Part model, mm, in its own coordinate system. A direction names the side the tool comes from. Give positions to 0.01 mm unless a question says otherwise; leave off trailing zeros. Order: outer loops, then holes, each group sorted by start corner. A loop starts at its lowest first (then second) coordinate and runs counter-clockwise, first axis right, second up. Notation, with made-up numbers: M 24.5,-4.75 L 40.5,-4.75 A23 cw 40.5,9.25 Z; hole C 11,4 d8. An arc over 180 degrees is marked long. Answer as a JSON object with one key per item and string values.
Autodesk Inventor part; units mm, degrees
ref_plane "YZ Plane" through (0, 0, 0) normal (1, 0, 0) x (0, 1, 0)
ref_plane "XZ Plane" through (0, 0, 0) normal (0, 1, 0) x (-1, 0, 0)
ref_plane "XY Plane" through (0, 0, 0) normal (0, 0, 1) x (1, 0, 0)
sketch "Sketch1" plane through (0, 0, 0) normal (0, 0, 1) x (1, 0, 0)
  line L0 (-27.5, 19) -> (27.5, 19)
  line L1 (27.5, 19) -> (27.5, -19)
  line L2 (27.5, -19) -> (-27.5, -19)
  line L3 (-27.5, -19) -> (-27.5, 19)
  line L4 (-27.5, 19) -> (27.5, -19) construction
  line L5 (27.5, 19) -> (-27.5, -19) construction
  point P0 (0, 0)
  dimension "d2" = 38
  dimension "d3" = 55
extrude "Extrusion1" add sketch "Sketch1" along normal mid plane 5
sketch "Sketch2" plane through (0, 0, 2.5) normal (0, 0, 1) x (1, 0, 0)
  line L0 (-27.5, -19) -> (27.5, -19)
  line L1 (27.5, -19) -> (27.5, 19)
  line L2 (27.5, 19) -> (-27.5, 19)
  line L3 (-27.5, 19) -> (-27.5, -19)
  point P0 (0, 0)
  point P1 (-15, 15)
  point P2 (15, 15)
  point P3 (-15, -15)
  point P4 (15, -15)
  point P5 (0, 0)
  point P6 (15.6, 0)
  point P7 (-15.6, 0)
  dimension "d4" = 15
  dimension "d5" = 15
  dimension "d36" = 30
  dimension "d43" = 30
  dimension "d50" = 15.6
  dimension "d57" = 15.6
hole "Hole1" at (-15.6, 0, 2.5) at (-15, 15, 2.5) at (15, 15, 2.5) at (15.6, 0, 2.5) at (15, -15, 2.5) at (-15, -15, 2.5) direction (0, 0, -1) diameter 2.5 end through all
sketch "Sketch3" plane through (0, 0, 2.5) normal (0, 0, 1) x (1, 0, 0)
  point P0 (0, 0)
  point P1 (0, 0)
hole "Hole2" at (0, 0, 2.5) direction (0, 0, -1) diameter 3.175 end through all
sketch "Sketch4" plane through (0, 0, 2.5) normal (0, 0, 1) x (1, 0, 0)
  line L0 (-27.5, 19) -> (-27.5, -19)
  line L1 (27.5, -19) -> (27.5, 19)
  point P0 (0, 0)
  point P1 (-22.5, 0)
  point P2 (22.5, 0)
  dimension "d76" = 5
  dimension "d77" = 5
  dimension "d89" = 22.5
hole "Hole3" at (-22.5, 0, 2.5) at (22.5, 0, 2.5) direction (0, 0, -1) diameter 2.459 end through all counterbore diameter 6 counterbore depth 1
properties part number "baseplate"
1. Which spindle directions (+Z, -Z, +X, -X, +Y, -Y) get a long thin tool onto all of the face, cutting with end or side? Do faces 1 (the cylindrical face through (25.43, 0.65, 1.99)), 2 (the flat face through (0, 4, 2.5)). Say none if no direction does.
Worked answers:
{"face 1": "+Z", "face 2": "+Z, +X, -X, +Y, -Y"}
2. Pin check, flat tip, straight feed: P1, Ø3.5, axis at x = -22.5, y = 0, coming from the +Z side. Stop position of the tip, or through.
Worked answers:
{"P1": "stops at z = 1.5"}
3. Probe line 1 along X through (y, z) = (0, -0.45); line 2 along X through (y, z) = (15, -0.4); line 3 along Y through (x, z) = (0, 0.2). List the from-to ranges inside material, lowest first.
Worked answers:
{"line 1": "x = -27.5 to -23.73, -21.27 to -16.85, -14.35 to -1.59, 1.59 to 14.35, 16.85 to 21.27, 23.73 to 27.5", "line 2": "x = -27.5 to -16.25, -13.75 to 13.75, 16.25 to 27.5", "line 3": "y = -19 to -1.59, 1.59 to 19"}
4. Cut at C-C on y = 15. Give the cut face in (x, z).
Worked answers:
{"outline": "M -27.5,-2.5 L -16.25,-2.5 L -16.25,2.5 L -27.5,2.5 Z; M -13.75,-2.5 L 13.75,-2.5 L 13.75,2.5 L -13.75,2.5 Z; M 16.25,-2.5 L 27.5,-2.5 L 27.5,2.5 L 16.25,2.5 Z"}
5. Cut at D-D on x = -22.5. Give the cut face in (y, z), plus the area to 3 significant figures.
Worked answers:
{"outline": "M -19,-2.5 L -1.23,-2.5 L -1.23,1.5 L -3,1.5 L -3,2.5 L -19,2.5 Z; M 1.23,-2.5 L 19,-2.5 L 19,2.5 L 3,2.5 L 3,1.5 L 1.23,1.5 Z", "area": "174 mm^2"}
6. Two-plate mould, pull along Y, no slides. Class faces 3 (the flat face through (0, 19, 0)), 4 (the flat face through (0, 4, -2.5)), 5 (the cylindrical face through (-15.845, 15.921, -0.035)), 6 (the cylindrical face through (-19.57, 0.65, 1.99)): +Y half, -Y half, draft (parallel to the pull), parting line (faces both ways), or undercut.
Worked answers:
{"face 3": "+Y half", "face 4": "draft", "face 5": "undercut", "face 6": "undercut"}
7. Cut at A-A on y = 0. State how many separate pieces and enclosed holes the cut face has, plus the area to 3 significant figures.
Worked answers:
{"separate pieces": "6", "enclosed holes": "0", "area": "202 mm^2"}
